Work out the finished part from the listing and answer in its coordinate system (mm). Face numbers are marked on the shaded views. A direction names the side the tool comes from. Round coordinates to 2 decimals unless told otherwise and drop trailing zeros. Order: outer loops, then holes, each group sorted by start corner. A loop starts at its lowest first (then second) coordinate and runs counter-clockwise, first axis right, second up.
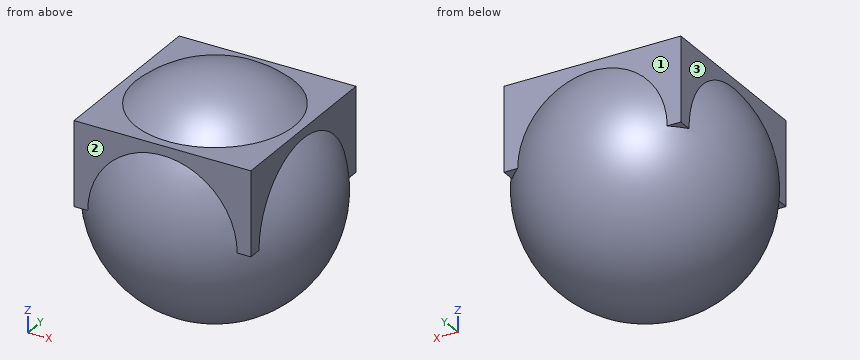
from build123d import *

# Parameters (mm, degrees)
F2_W     = 42
F2_H     = 42
F3_DEPTH = 20


with BuildPart() as f1:
    # F0 (on Front) → F1 (revolve)
    with BuildSketch(Plane.XZ):
        with BuildLine():
            Line((0, -27.5), (0, 27.5))
            ThreePointArc((0, 27.5), (-27.5, 0), (0, -27.5))
        make_face()
    revolve(axis=Axis((0, 0, 0.613028), (0, 0, 1)))

    # F2 (on Top) → F3 (join)
    with BuildSketch(Plane.XY):
        Rectangle(F2_W, F2_H)
    extrude(amount=F3_DEPTH)


solid = f1.part
Item 1: Find section A-A (z = 15.5). Write down the section's boundary in (x, y), plus the area to 3 significant figures.
Item 2: Find the intervals of material crossed by line 1 along X through (y, z) = (-16, 18); line 2 along X through (y, z) = (-4.5, 23), in increasing order.
Item 3: A tool of negligible diameter and unlimited length cuts with its end or side. For the marked faces 1, 2 and 3, from which of +Z, -Z, +X, -X, +Y, -Y can it reach the whole face along a straight path? Write none if from no direction.
Item 4: Given pin 1 (22 mm diameter, centred on y = 2, z = 14.5, fed in from -X); pin 2 (22 mm diameter, centred on x = -3.5, z = 7, fed in from +Y); pin 3 (8 mm diameter, centred on x = -7.5, z = -13, fed in from -Y); pin 4 (16 mm diameter, centred on x = 10.5, z = 8.5, fed in from -Y), each flat-ended and moving along its own axis, determine where each tip first touches the part or whether it passes through.
Item 5: Find section C-C (x = 5). Write down the section's boundary in (y, z).
Item 6: Find section B-B (y = 20). Write down the section's boundary in (x, z).
Item 7: Find section D-D (z = 6.5). Write down the section's boundary in (x, y).
Model answer:
1. outline: (-21, -21) - (-8.66, -21) arc R22.72 ccw to (8.66, -21) - (21, -21) - (21, -8.66) arc R22.72 ccw to (21, 8.66) - (21, 21) - (8.66, 21) arc R22.72 ccw to (-8.66, 21) - (-21, 21) - (-21, 8.66) arc R22.72 ccw to (-21, -8.66) - close
1. area: 1,840 mm2
2. line 1: x = -21 to 21
2. line 2: x = -14.39 to 14.39
3. face 1: +Z, +Y
3. face 2: +Z, -Y
3. face 3: +Z, -X
4. pin 1: stops at x = -27.26
4. pin 2: stops at y = 27.5
4. pin 3: stops at y = -25.2
4. pin 4: stops at y = -26.94
5. outline: (-21, 17.04) arc R27.04 ccw (long way) to (21, 17.04) - (21, 20) - (18.2, 20) arc R27.04 ccw to (-18.2, 20) - (-21, 20) - close
6. outline: (-21, 0) - (-18.87, 0) arc R18.87 ccw to (18.87, 0) - (21, 0) - (21, 20) - (-21, 20) - close
7. outline: (-21, -21) - (-16.52, -21) arc R26.72 ccw to (16.52, -21) - (21, -21) - (21, -16.52) arc R26.72 ccw to (21, 16.52) - (21, 21) - (16.52, 21) arc R26.72 ccw to (-16.52, 21) - (-21, 21) - (-21, 16.52) arc R26.72 ccw to (-21, -16.52) - close
